Input: dimensioned drawing with shaded views. Units: mm. Origin: part minimum x, y, z. A direction names the side the tool comes from. Round coordinates to 2 decimals unless told otherwise and drop trailing zeros. Loops run counter-clockwise (first coordinate to the right, second up) from the corner with the lowest first, then second, coordinate; pieces in that order, holes last. Notation, with made-up numbers: M 57.25,-9.75 L 61.25,-9.75 A20 cw 61.25,3.25 Z; hole C 44,82.5 d11. An arc over 180 degrees is marked long. One line per item, written item: value.
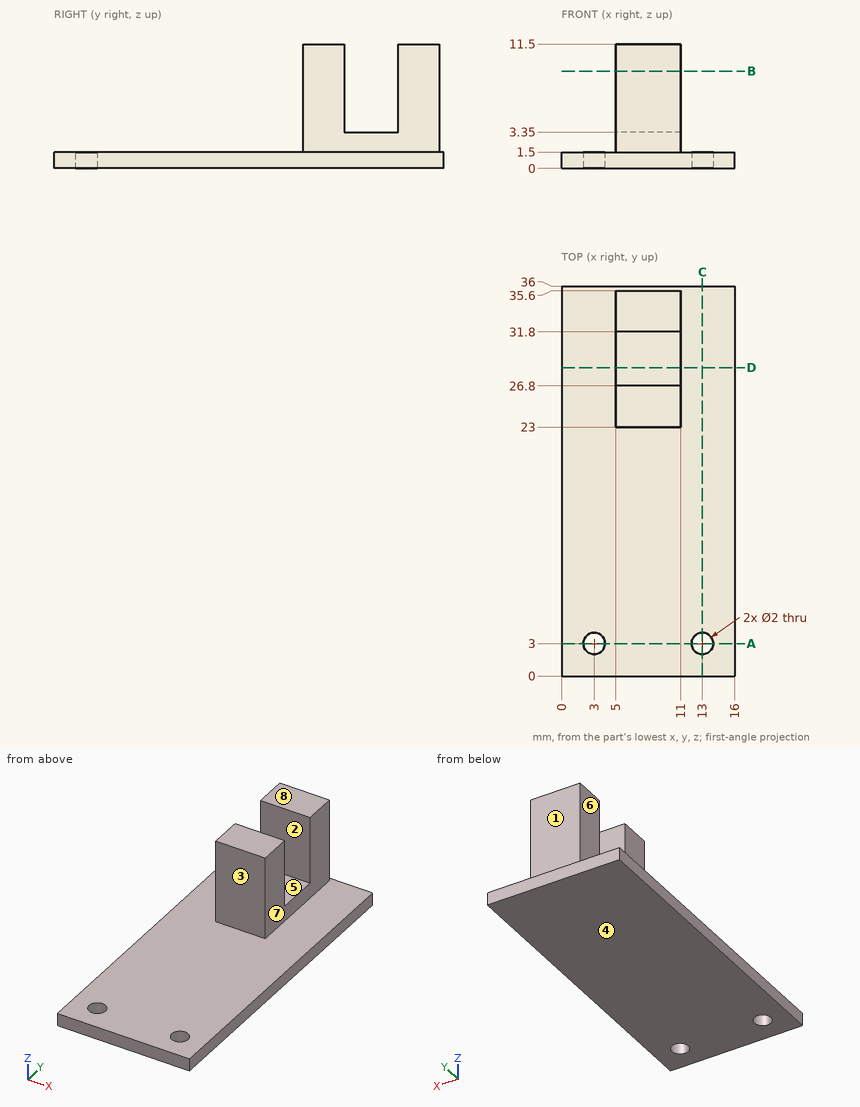
1. Reachability of the marked faces 5, 6, 7 and 8 from +Z, -Z, +X, -X, +Y, -Y: full face, straight path, thin tool, end or side. Return the list, or none.
Report:
face 5: +Z, +X, -X
face 6: +Z, -X, +Y, -Y
face 7: +Z, +X, +Y, -Y
face 8: +Z, +X, -X, +Y, -Y
2. Section query B-B (z = 9). Return the cut outline in (x, y), and give its area (3 significant figures).
Report:
outline: M 5,23 L 11,23 L 11,26.8 L 5,26.8 Z; M 5,31.8 L 11,31.8 L 11,35.6 L 5,35.6 Z
area: 45.6 mm2
3. Ray query, line 1 (X direction, y = 3, z = 0.4); line 2 (Z direction, x = 13.25, y = 14); line 3 (Z direction, x = 9, y = 28). Return the intervals inside material, ascending. Write a range as [from, to].
Report:
line 1: x = [0, 2], [4, 12], [14, 16]
line 2: z = [0, 1.5]
line 3: z = [0, 3.35]
4. Section query C-C (x = 13). Return the cut outline in (y, z).
Report:
outline: M 0,0 L 2,0 L 2,1.5 L 0,1.5 Z; M 4,0 L 36,0 L 36,1.5 L 4,1.5 Z
5. Section query A-A (y = 3). Return the cut outline in (x, z), and give its area (3 significant figures).
Report:
outline: M 0,0 L 2,0 L 2,1.5 L 0,1.5 Z; M 4,0 L 12,0 L 12,1.5 L 4,1.5 Z; M 14,0 L 16,0 L 16,1.5 L 14,1.5 Z
area: 18.0 mm2
6. Section query D-D (y = 28.5). Return the cut outline in (x, z).
Report:
outline: M 0,0 L 16,0 L 16,1.5 L 11,1.5 L 11,3.35 L 5,3.35 L 5,1.5 L 0,1.5 Z
7. Pull-direction query (Y, two-part tool) for the marked faces 1, 2, 3 and 4; classes: released by +Y, released by -Y, zero draft, split by the parting line, or undercut.
Report:
face 1: released by +Y
face 2: undercut
face 3: released by -Y
face 4: zero draft
8. Pin query (flat end, axial travel): pin 1 (5 mm diameter, centred on x = 9, z = 6, fed in from -Y); pin 2 (6.5 mm diameter, centred on x = 7.5, z = 6.5, fed in from +Y); pin 3 (2.5 mm diameter, centred on x = 13, y = 3, fed in from +Z); pin 4 (1.8 mm diameter, centred on x = 3, y = 3, fed in from +Z). Return the tip coordinate at first contact, or that it passes through.
Report:
pin 1: stops at y = 23
pin 2: stops at y = 35.6
pin 3: stops at z = 1.5
pin 4: passes through
